Answer from the drawing. Dimensions are ordinates in mm from the lowest x, y and z of the part. Coordinates: 2 decimals unless noted, no trailing zeros. Write each loop counter-clockwise with the first axis right and the second up, starting at its lowest first coordinate (ties: lowest second). Pieces come first, ordered by that corner, then holes. Notation, with made-up numbers: (5, -35) - (16, -35) arc R17 cw to (16, -25) - close; hole circle Ø2 at (20, -28.5). An arc over 180 degrees is marked (long way). Use CSV: the item, a comma, the result in double quotes. Start each with the question number.
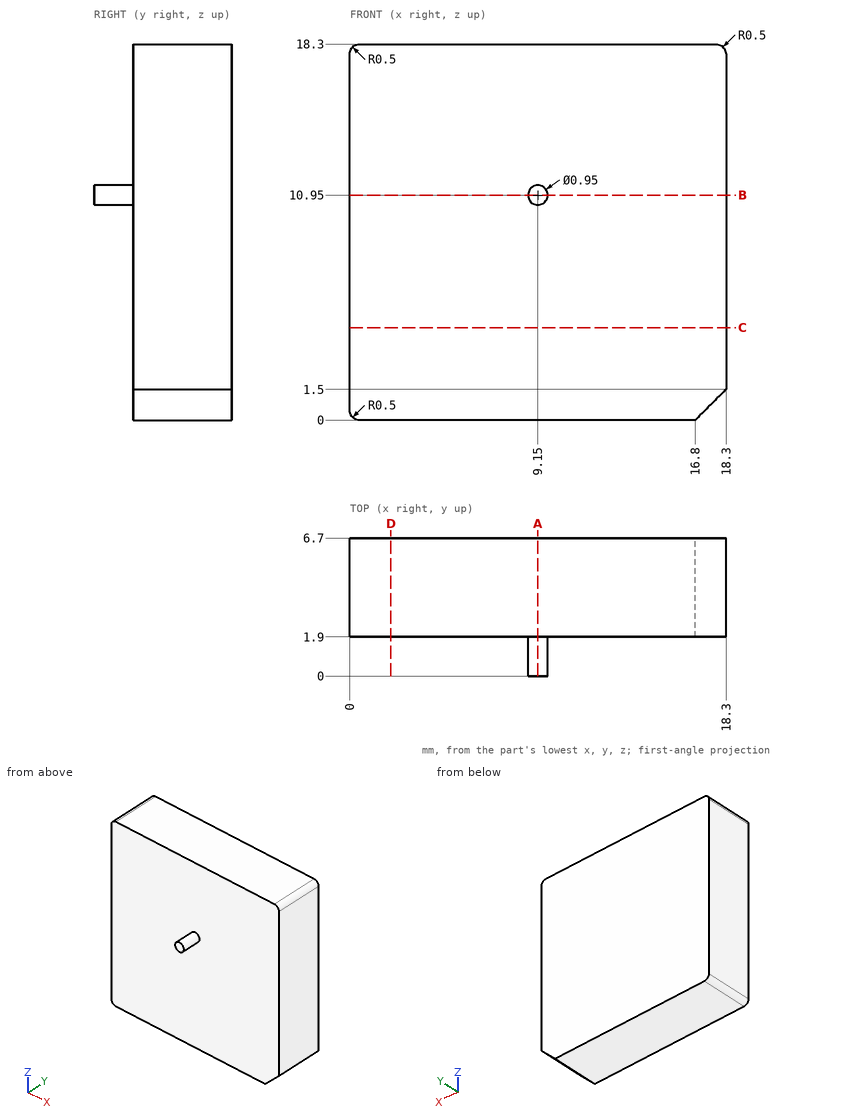
Item 1: A cutting plane is placed at A-A (x = 9.15). Determine the outline of the cut face in (y, z) (3 decimals).
Item 2: A cutting plane is placed at C-C (z = 4.5). Determine the outline of the cut face in (x, y).
Item 3: A cutting plane is placed at D-D (x = 2). Determine the outline of the cut face in (y, z).
Item 4: A cutting plane is placed at B-B (z = 10.95). Determine the outline of the cut face in (x, y) (3 decimals), then the cut area to 3 significant figures.
Item 5: This flat-tipped pin is pushed along its axis until it touches: pin 1 (4 mm diameter, centred on x = 6, z = 2, fed in from -Y). Where does it stop, or does it pass through?
Item 6: A straight line is drawn through the part: probe 1 along Y at (x, z) = (15, 3.5). Find the intervals that lie inside material, in ascending order. Write a range as [from, to].
Calculated:
1,outline,"(0, 10.475) - (1.9, 10.475) - (1.9, 0) - (6.7, 0) - (6.7, 18.3) - (1.9, 18.3) - (1.9, 11.425) - (0, 11.425) - close"
2,outline,"(0, 1.9) - (18.3, 1.9) - (18.3, 6.7) - (0, 6.7) - close"
3,outline,"(1.9, 0) - (6.7, 0) - (6.7, 18.3) - (1.9, 18.3) - close"
4,outline,"(0, 1.9) - (8.675, 1.9) - (8.675, 0) - (9.625, 0) - (9.625, 1.9) - (18.3, 1.9) - (18.3, 6.7) - (0, 6.7) - close"
4,area,"89.6 mm²"
5,pin 1,"stops at y = 1.9"
6,probe 1,"y = [1.9, 6.7]"
